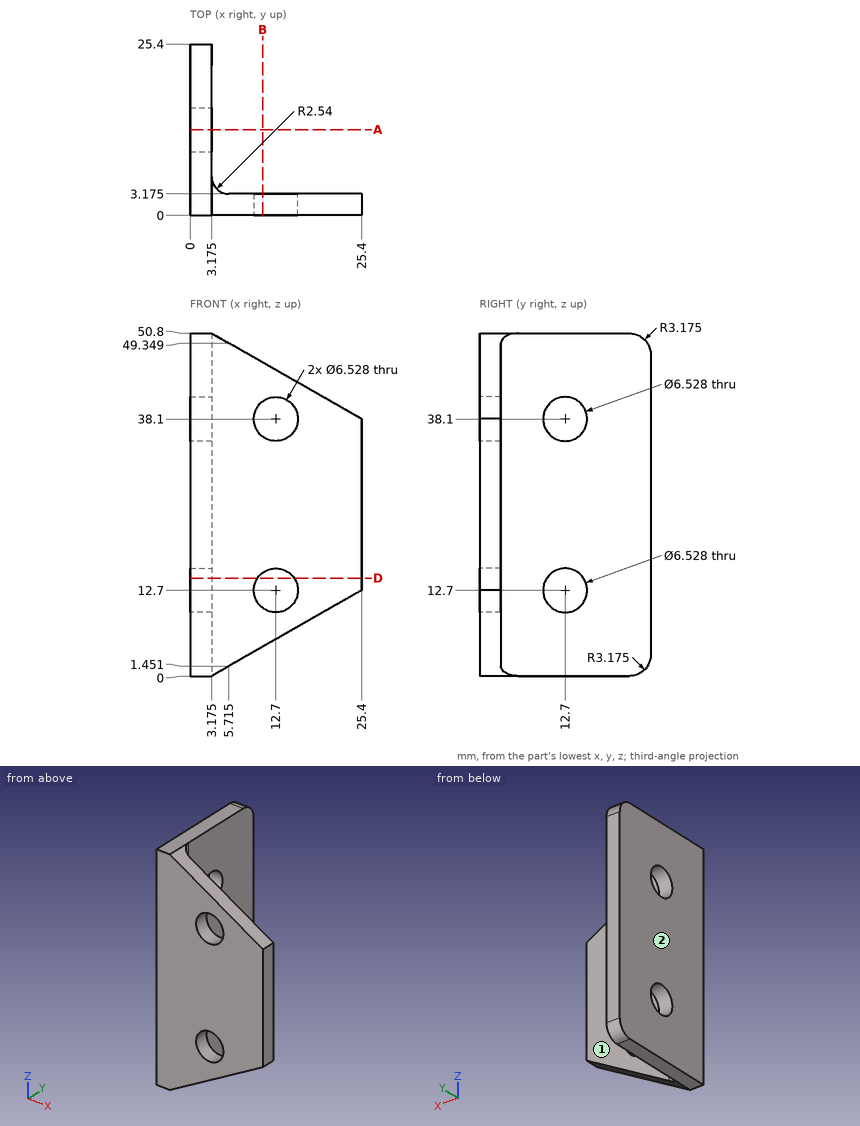
Answer from the drawing. Dimensions are ordinates in mm from the lowest x, y and z of the part. A direction names the side the tool comes from. Round coordinates to 2 decimals unless told otherwise and drop trailing zeros. Loops run counter-clockwise (first coordinate to the right, second up) from the corner with the lowest first, then second, coordinate; pieces in that order, holes last.
Q1. Section A-A on y = 12.7 is taken. Write down the section's boundary in (x, z) (1 decimal).
Q2. Which of the six approach directions +Z, -Z, +X, -X, +Y, -Y give full straight-line access (tool end or side, diameter ignored) to the marked faces 1 and 2?
Q3. Each of these flat-tipped pins is pushed along its axis until it touches: pin 1 (8.5 mm diameter, centred on y = 12.7, z = 12.7, fed in from +X) (3 decimals); pin 2 (10 mm diameter, centred on x = 17, z = 36, fed in from +Y) (3 decimals); pin 3 (10.5 mm diameter, centred on y = 12.7, z = 38.1, fed in from -X). Where does it stop, or does it pass through?
Q4. Consider probe 1 along Z at (x, y) = (12.7, 2.2) (1 decimal); probe 2 along X at (y, z) = (14.75, 46) (1 decimal); probe 3 along Y at (x, z) = (0.6, 12.7). Determine where each line is inside the solid, lowest interval first.
Q5. Section B-B on x = 10.75 is taken. Write down the section's boundary in (y, z) (1 decimal).
Q6. Section D-D on z = 14.5 is taken. Write down the section's boundary in (x, y) (1 decimal).
Output:
1. outline: (0, 0) - (3.2, 0) - (3.2, 9.4) - (0, 9.4) - close; (0, 16) - (3.2, 16) - (3.2, 34.8) - (0, 34.8) - close; (0, 41.4) - (3.2, 41.4) - (3.2, 50.8) - (0, 50.8) - close
2. face 1: +Z, -Z, +X, +Y
2. face 2: +Z, -Z, -X, +Y, -Y
3. pin 1: stops at x = 3.175
3. pin 2: stops at y = 3.175
3. pin 3: stops at x = 0
4. probe 1: z = 5.4 to 9.4, 16 to 34.8, 41.4 to 45.4
4. probe 2: x = 0 to 3.2
4. probe 3: y = 0 to 9.44, 15.96 to 25.4
5. outline: (0, 4.3) - (3.2, 4.3) - (3.2, 10.1) - (0, 10.1) - close; (0, 15.3) - (3.2, 15.3) - (3.2, 35.5) - (0, 35.5) - close; (0, 40.7) - (3.2, 40.7) - (3.2, 46.5) - (0, 46.5) - close
6. outline: (0, 0) - (10, 0) - (10, 3.2) - (5.7, 3.2) arc R2.5 cw to (3.2, 5.7) - (3.2, 10) - (0, 10) - close; (0, 15.4) - (3.2, 15.4) - (3.2, 25.4) - (0, 25.4) - close; (15.4, 0) - (25.4, 0) - (25.4, 3.2) - (15.4, 3.2) - close
